Geometry check sheet. Reference: the model listing, model coordinates, mm. Round coordinates to 2 decimals unless told otherwise and drop trailing zeros. Write each loop counter-clockwise with the first axis right and the second up, starting at its lowest first coordinate (ties: lowest second). Pieces come first, ordered by that corner, then holes. Notation, with made-up numbers: (46, 73) -> (85, 73) arc R7 cw to (85, 85) -> close; hole circle Ø1 at (7, -35). An arc over 180 degrees is marked (long way). One line per question, with ' | ' between items.
```python
from build123d import *

# Parameters (mm, degrees)
SKETCH1_R           = 12.5
BOSS_EXTRUDE1_DEPTH = 5.953125
SKETCH2_R           = 2.7781
CUT_EXTRUDE1_DEPTH  = 5.953125
FILLET1_R           = 1


with BuildPart() as part:
    # Sketch1 → Boss-Extrude1 (new body)
    with BuildSketch(Plane(origin=(0, 0, 0), x_dir=(1, 0, 0), z_dir=(0, 1, 0))):
        Circle(SKETCH1_R)
    extrude(amount=BOSS_EXTRUDE1_DEPTH)

    # Sketch2 → Cut-Extrude1 (cut)
    with BuildSketch(Plane(origin=(0, 5.953125, 0), x_dir=(1, 0, 0), z_dir=(0, 1, 0))):
        Circle(SKETCH2_R)
    extrude(amount=-CUT_EXTRUDE1_DEPTH, mode=Mode.SUBTRACT)

    # Fillet1
    fillet1_edges = [part.edges().sort_by_distance(p)[0] for p in [
        (-12.5, 0, 0),
        (-12.5, 5.953125, 0),
        (-2.7781, 5.953125, 0),
        (-2.7781, 0, 0),
    ]]
    fillet(fillet1_edges, radius=FILLET1_R)


solid = part.part
```
(1) Sectioned sample at A-A on x = 0. Record the cut outline in (y, z).
Resolved:
outline: (0, -11.5) arc R1 ccw to (1, -12.5) -> (4.95, -12.5) arc R1 ccw to (5.95, -11.5) -> (5.95, -3.78) arc R1 ccw to (4.95, -2.78) -> (1, -2.78) arc R1 ccw to (0, -3.78) -> close; (0, 3.78) arc R1 ccw to (1, 2.78) -> (4.95, 2.78) arc R1 ccw to (5.95, 3.78) -> (5.95, 11.5) arc R1 ccw to (4.95, 12.5) -> (1, 12.5) arc R1 ccw to (0, 11.5) -> close
(2) Sectioned sample at B-B on z = 0. Record the cut outline in (x, y).
Resolved:
outline: (-12.5, 1) arc R1 ccw to (-11.5, 0) -> (-3.78, 0) arc R1 ccw to (-2.78, 1) -> (-2.78, 4.95) arc R1 ccw to (-3.78, 5.95) -> (-11.5, 5.95) arc R1 ccw to (-12.5, 4.95) -> close; (2.78, 1) arc R1 ccw to (3.78, 0) -> (11.5, 0) arc R1 ccw to (12.5, 1) -> (12.5, 4.95) arc R1 ccw to (11.5, 5.95) -> (3.78, 5.95) arc R1 ccw to (2.78, 4.95) -> close
(3) Draft check along X on faces 1 (the cylindrical face through (-2.205, 3.004, 1.69)), 2 (the flat face through (-3, 5.953, -3)), 3 (the cylindrical face through (11.923, 2.949, -3.755)). Enter one of: +X half, -X half, draft (parallel to the pull), parting line (faces both ways), or undercut.
Resolved:
face 1: undercut | face 2: draft | face 3: parting line
(4) Material ranges on line 1 (X direction, y = 1.9, z = 0); line 2 (Z direction, x = 1, y = 3.2), recorded low to high.
Resolved:
line 1: x = -12.5 to -2.78, 2.78 to 12.5 | line 2: z = -12.46 to -2.59, 2.59 to 12.46
(5) Go/stop test with flat-tipped pins: pin 1 (1.5 mm diameter, centred on y = 4.5, z = -10, fed in from +X); pin 2 (4 mm diameter, centred on x = -8, z = 0.5, fed in from -Y); pin 3 (1 mm diameter, centred on y = 5, z = 2.5, fed in from +X); pin 4 (3 mm diameter, centred on y = 3.5, z = -5, fed in from -X). Record where each tip stops, or that it passes through.
Resolved:
pin 1: stops at x = 8.41 | pin 2: stops at y = 0 | pin 3: stops at x = 12.34 | pin 4: stops at x = -12
(6) Sectioned sample at C-C on y = 1.7. Record the cut outline in (x, z), then the cut area to 3 significant figures.
Resolved:
outline: circle Ø25 at (0, 0); hole circle Ø5.56 at (0, 0) | area: 467 mm2
